Answer from the drawing. Dimensions are ordinates in mm from the lowest x, y and z of the part. A direction names the side the tool comes from. Coordinates: 2 decimals unless noted, no trailing zeros. Order: outer loops, then holes, each group sorted by start corner. A loop starts at its lowest first (then second) coordinate and runs counter-clockwise, first axis right, second up. Notation, with made-up numbers: M -9.75,-38.5 L 43.25,-38.5 A5 ccw 43.25,-29.5 Z; hole C -13,-19 d1. An arc over 180 degrees is marked long. One line per question, with ' | ' between items. Start each with the question number.
1) Find section B-B, the plane x = 7.5. Write down the section's boundary in (y, z).
2) Find section D-D, the plane z = 10. Write down the section's boundary in (x, y), plus the area to 4 significant figures.
3) Consider probe 1 along Y at (x, z) = (0.65, 7.5); probe 2 along X at (y, z) = (11.75, 8). Determine where each line is inside the solid, lowest interval first.
4) A tool of negligible diameter and unlimited length cuts with its end or side. For the marked faces 1 and 2, from which of +Z, -Z, +X, -X, +Y, -Y can it reach the whole face along a straight path? Write none if from no direction.
5) Find section A-A, the plane z = 7.5. Write down the section's boundary in (x, y), plus the area to 4 significant figures.
6) Given P1, Ø4, axis at y = 10, z = 4.5, coming from the +X side; P2, Ø2.5, axis at x = 7.5, z = 7.5, coming from the -Y side; P3, Ø2, axis at y = 2, z = 7.5, coming from the +X side, each flat-ended and moving along its own axis, determine where each tip first touches the part or whether it passes through.
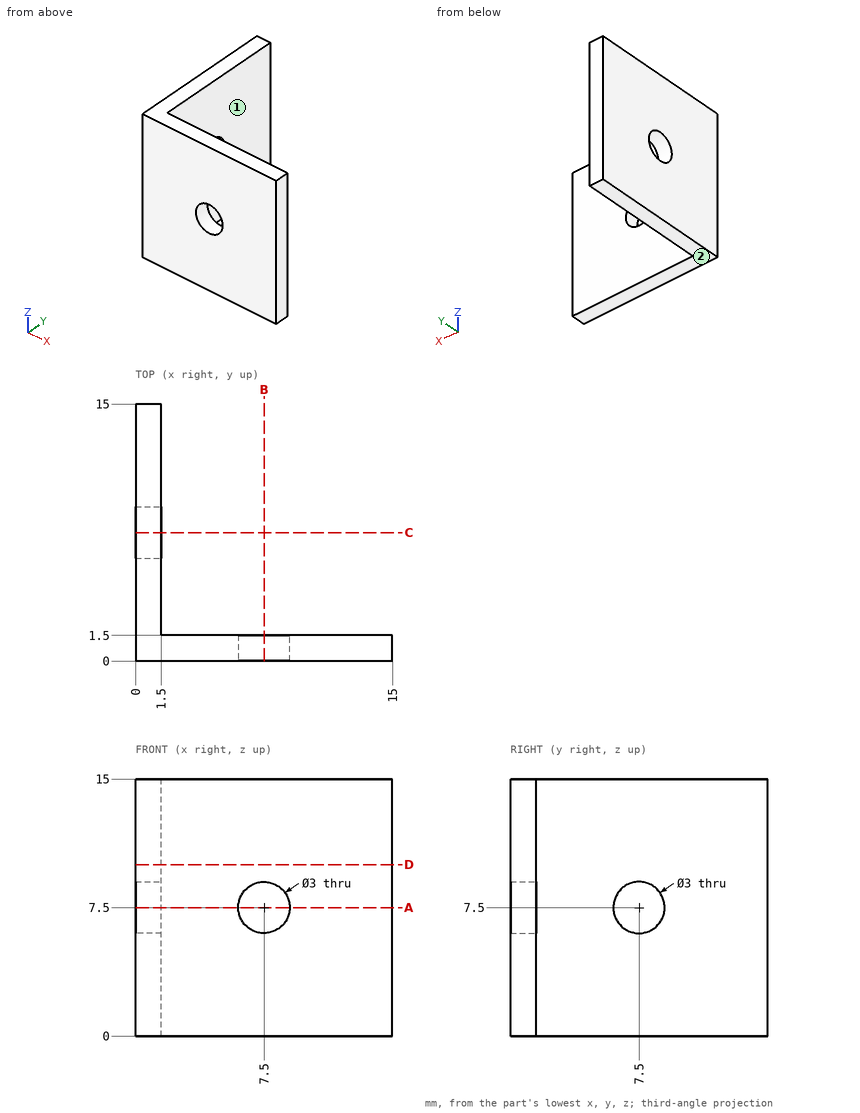
Report:
1) outline: M 0,0 L 1.5,0 L 1.5,6 L 0,6 Z; M 0,9 L 1.5,9 L 1.5,15 L 0,15 Z
2) outline: M 0,0 L 15,0 L 15,1.5 L 1.5,1.5 L 1.5,15 L 0,15 Z | area: 42.75 mm^2
3) probe 1: y = 0 to 6, 9 to 15 | probe 2: x = 0 to 1.5
4) face 1: +Z, -Z, +X, +Y | face 2: -Z, +X, -X, +Y, -Y
5) outline: M 0,0 L 6,0 L 6,1.5 L 1.5,1.5 L 1.5,6 L 0,6 Z; M 0,9 L 1.5,9 L 1.5,15 L 0,15 Z; M 9,0 L 15,0 L 15,1.5 L 9,1.5 Z | area: 33.75 mm^2
6) P1: stops at x = 1.5 | P2: passes through | P3: stops at x = 15
